Read the model definition and answer for the solid it produces. Units are mm, in the model's axes. Face numbers are marked on the shaded views. A direction names the side the tool comes from. Give positions to 0.01 mm unless a question says otherwise; leave off trailing zeros. Loops run counter-clockwise (first coordinate to the right, second up) from the corner with the lowest first, then second, coordinate; pieces in that order, holes last. Notation, with made-up numbers: (45.25, 9) -> (87.25, 9) arc R16 cw to (87.25, 35) -> close; hole circle Ø6 at (49.25, 63.25). An arc over 180 degrees is marked (long way). Return JSON: item names as keys, results as strings. Group by question number.
from build123d import *

# Parameters (mm, degrees)
F2_W     = 2.503898
F2_H     = 5.537905
F3_DEPTH = 2


with BuildPart() as f1:
    # F0 (on Front) → F1 (revolve)
    with BuildSketch(Plane.XZ):
        with BuildLine():
            Line((0, 70), (0, 0))
            Line((0, 0), (5, 0))
            Line((5, 0), (5, 20))
            Line((5, 20), (20, 20))
            ThreePointArc((20, 20), (14.662927, 30), (20, 40))
            Line((20, 40), (5, 40))
            Line((5, 40), (5, 70))
            Line((5, 70), (0, 70))
        make_face()
    revolve(axis=Axis((0, 0, 35), (0, 0, 1)))

    # F2 (on face) → F3 (join)
    with BuildSketch(Plane.XY.offset(40)):
        with Locations((1.251949, -13.775359)):
            Rectangle(F2_W, F2_H)
    extrude(amount=F3_DEPTH)


solid = f1.part
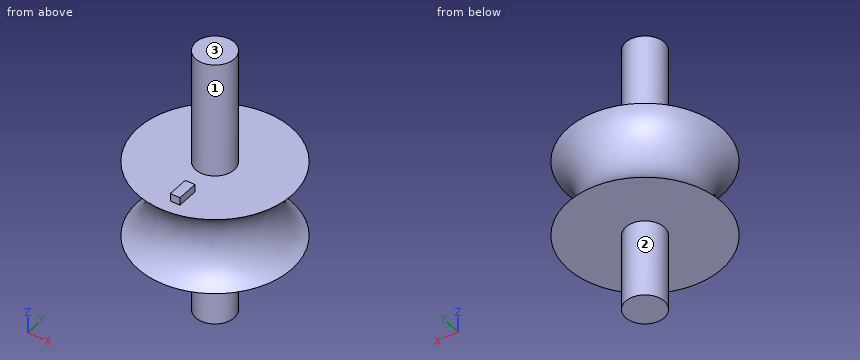
1. Which of the six approach directions +Z, -Z, +X, -X, +Y, -Y give full straight-line access (tool end or side, diameter ignored) to the marked faces 1, 2 and 3?
2. Section A-A on y = 0 is taken. Determine the outline of the cut face in (x, z), then the cut area to 3 significant figures.
3. Flat-ended cylindrical pins translate along their axes: pin 1 Ø0.6 at (y, z) = (-12.5, 40.5) entering from -X; pin 2 Ø0.6 at (x, z) = (1.5, 40.5) entering from +Y; pin 3 Ø2 at (x, y) = (-6.5, 0.5) entering from -Z; pin 4 Ø12 at (x, y) = (3.5, -4.5) entering from -Z. Find the tip coordinate at first contact, or state that the pin passes through.
4. Straight lines are drawn through the part: line 1 (Z direction, x = 4.5, y = 9.5); line 2 (Z direction, x = 12, y = 10); line 3 (Z direction, x = -11, y = 11). For each, find the intervals that lie inside material, in ascending order. Write a range as from..to.
5. Section B-B on z = 24.5 is taken. Determine the outline of the cut face in (x, y).
Completed:
{
 "1": {"face 1": "+Z", "face 2": "-Z", "face 3": "+Z, +X, -X, +Y, -Y"},
 "2": {"outline": "(-20, 20) -> (-5, 20) -> (-5, 0) -> (5, 0) -> (5, 20) -> (20, 20) arc R12.04 cw to (20, 40) -> (5, 40) -> (5, 70) -> (-5, 70) -> (-5, 40) -> (-20, 40) arc R12.04 cw to start", "area": "1,150 mm²"},
 "3": {"pin 1": "stops at x = 0", "pin 2": "stops at y = 4.85", "pin 3": "stops at z = 20", "pin 4": "stops at z = 0"},
 "4": {"line 1": "z = 20..40", "line 2": "z = 20..25.3, 34.7..40", "line 3": "z = 20..25.45, 34.55..40"},
 "5": {"outline": "circle Ø31.99 at (0, 0)"}
}
